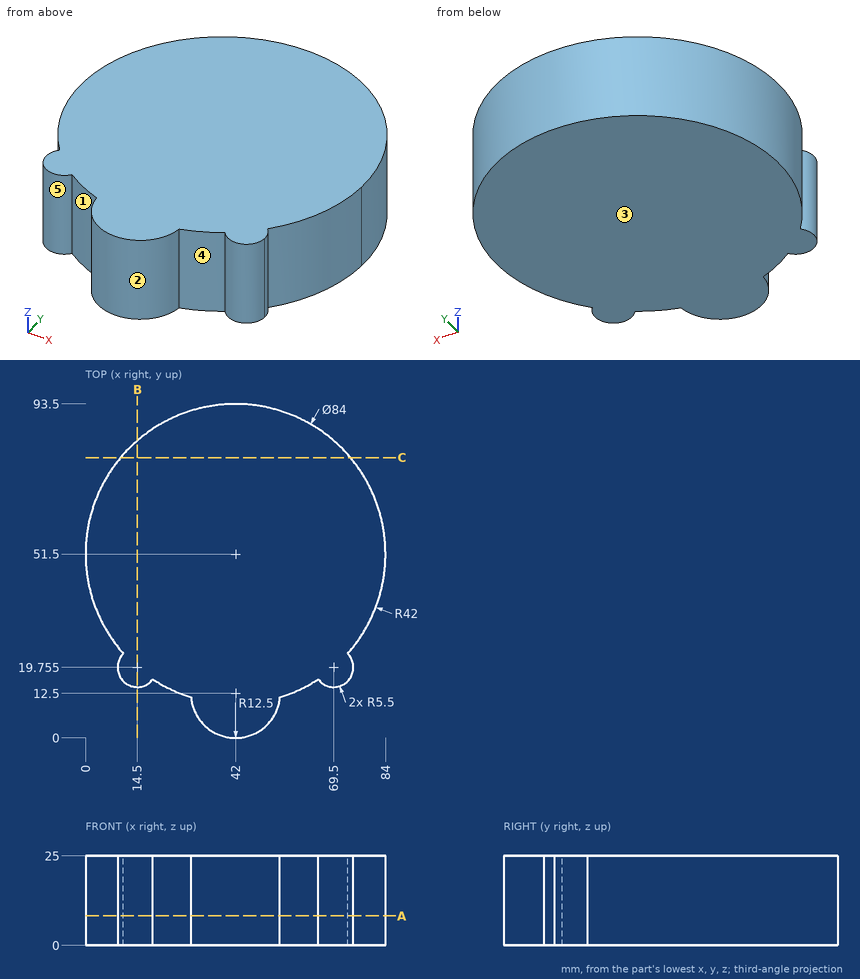
Can you work these out from the drawing? Everything is in mm from the part's minimum corner. A direction names the side the tool comes from. Give positions to 0.01 mm unless a question says otherwise; leave off trailing zeros. Write each loop counter-clockwise with the first axis right and the second up, starting at its lowest first coordinate (ties: lowest second). Pieces come first, ordered by that corner, then holes. Notation, with made-up numbers: M 9,-14.75 L 31,-14.75 A27 cw 31,23.25 Z; hole C 41.5,-1.5 d9. An arc over 180 degrees is marked long. Answer in a Markdown table with one row per item. Add a question column.
Item 1: We'd pull the mould along X, two halves only. Please class the marked faces 1, 2 and 3: released by +X, released by -X, zero draft, split by the parting line, or undercut.
Item 2: Imagine slicing it at B-B, the plane x = 14.5. Write out the boundary of the cut face in (y, z) (3 decimals), plus the area to 3 significant figures.
Item 3: Please list where these lines run through material, in increasing order: L1, parallel to X at y = 21.5, z = 11.25; L2, parallel to X at y = 71, z = 13.5; L3, parallel to Y at x = 16.5, z = 11.
Item 4: Imagine slicing it at A-A, the plane z = 8.25. Write out the boundary of the cut face in (x, y) (1 decimal), plus the area to 3 significant figures.
Item 5: Imagine slicing it at C-C, the plane y = 78.5. Write out the boundary of the cut face in (x, z).
Item 6: On a 3-axis mill with a long thin cutter (end or side, diameter ignored), from which of +Z, -Z, +X, -X, +Y, -Y can I reach the whole of each face in a straight line? I mean the marked faces 4 and 5. Say none if no direction works.
Item 7: For pin 1 Ø5 at (x, z) = (33, 16) entering from +Y; pin 2 Ø2 at (x, z) = (16.5, 3.5) entering from -Y; pin 3 Ø3 at (x, z) = (56.5, 20) entering from -Y, each with a flat end and sliding along its axis, tell me the tip position at first contact or that it passes through.
Evaluation:
| question | item | result |
|---|---|---|
| 1 | face 1 | undercut |
| 1 | face 2 | split by the parting line |
| 1 | face 3 | zero draft |
| 2 | outline | M 14.255,0 L 83.245,0 L 83.245,25 L 14.255,25 Z |
| 2 | area | 1,720 mm² |
| 3 | L1 | x = 9.28 to 74.72 |
| 3 | L2 | x = 4.8 to 79.2 |
| 3 | L3 | y = 14.63 to 84.87 |
| 4 | outline | M 10.6,23.6 A5.5 ccw long 18.9,16.4 A42 ccw 29.5,11.4 A12.5 ccw 54.5,11.4 A42 ccw 65.1,16.4 A5.5 ccw long 73.4,23.6 A42 ccw long Z |
| 4 | area | 5,830 mm² |
| 5 | outline | M 9.83,0 L 74.17,0 L 74.17,25 L 9.83,25 Z |
| 6 | face 4 | +Z, -Z, -Y |
| 6 | face 5 | +Z, -Z |
| 7 | pin 1 | stops at y = 92.99 |
| 7 | pin 2 | stops at y = 14.35 |
| 7 | pin 3 | stops at y = 11.56 |
